```python
from build123d import *

# Parameters (mm, degrees)
SKETCH1_W           = 6
SKETCH1_H           = 6
BOSS_EXTRUDE1_DEPTH = 5
CUT_EXTRUDE5_DEPTH  = 3
CUT_EXTRUDE6_DEPTH  = 3


with BuildPart() as part:
    # Sketch1 → Boss-Extrude1 (new body)
    with BuildSketch(Plane(origin=(0, 0, 0), x_dir=(1, 0, 0), z_dir=(0, 1, 0))):
        Rectangle(SKETCH1_W, SKETCH1_H)
    extrude(amount=BOSS_EXTRUDE1_DEPTH)

    # Sketch8 → Cut-Extrude5 (cut)
    with BuildSketch(Plane.XY.offset(3)):
        Polygon((3, 3), (0, 1.5), (0, 3), (-3, 5), (3, 5), align=None)
    extrude(amount=-CUT_EXTRUDE5_DEPTH, mode=Mode.SUBTRACT)

    # Sketch9 → Cut-Extrude6 (cut)
    with BuildSketch(Plane(origin=(0, 0, -3), x_dir=(-1, 0, 0), z_dir=(0, 0, -1))):
        Polygon((-3, 5), (-3, 3), (0, 1.5), (3, 0), (3, 5), align=None)
    extrude(amount=-CUT_EXTRUDE6_DEPTH, mode=Mode.SUBTRACT)


solid = part.part
```
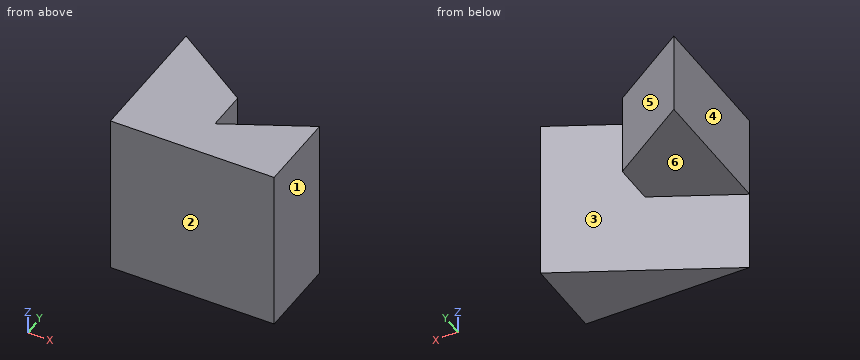
Model file for the job. Use its own axes, mm. Face numbers are marked on the shaded views. A direction names the side the tool comes from. Coordinates: 2 decimals unless noted, no trailing zeros. Order: outer loops, then holes, each group sorted by start corner. A loop starts at its lowest first (then second) coordinate and runs counter-clockwise, first axis right, second up. Notation, with made-up numbers: M 80.5,72 L 101.5,72 A26 cw 101.5,107 Z; hole C 70.25,-7.75 d7. An arc over 180 degrees is marked long. Answer as CSV lines item,"result".
(1) Flat gauge pins, fed straight in: pin 1 (2 mm diameter, centred on x = -0.5, z = 1, fed in from +Y); pin 2 (1.5 mm diameter, centred on y = 4, z = -2.5, fed in from +X). Where does each tip first touch, or does it go through?
Geometry says:
pin 1,"stops at y = 4"
pin 2,"passes through"
(2) Band-saw the part on D-D, the plane y = 3.1. List the corners of the cut face in (x, z).
Geometry says:
outline,"M -3,0 L -0.15,0 L -0.15,3 L -3,3 Z"
(3) Pull direction X, two halves, no side cores. Call the marked faces 1, 2, 3 and 4: +X half, -X half, draft (parallel to the pull), parting line (faces both ways), or undercut.
Geometry says:
face 1,"+X half"
face 2,"draft"
face 3,"undercut"
face 4,"-X half"
(4) Band-saw the part on A-A, the plane y = 2.4. List the corners of the cut face in (x, z).
Geometry says:
outline,"M -3,0 L 0,0 L 0,3 L -3,3 Z; M 1.8,-3 L 3,-3 L 3,3 L 1.8,3 Z"
(5) Band-saw the part on C-C, the plane x = -0.5. List the corners of the cut face in (y, z).
Geometry says:
outline,"M 0,-3 L 1.25,-3 L 1.25,0 L 3.33,0 L 3.33,3 L 0,3 Z"
(6) Band-saw the part on B-B, the plane z = 0.2. List the corners of the cut face in (x, y), then the cut area to 4 significant figures.
Geometry says:
outline,"M -3,0 L 3,0 L 3,3 L 0,1.5 L 0,3 L -3,5 Z"
area,"18.75 mm2"
(7) Wall check: line 1 along Z through (x, y) = (-0.25, 2.05); line 2 along Y through (x, z) = (0, -1); line 3 along Y through (x, z) = (2.5, 2.5). Give the ranges that are in metal, low to high.
Geometry says:
line 1,"z = 0 to 3"
line 2,"y = 0 to 1.5"
line 3,"y = 0 to 2.75"
(8) 3-axis set-ups, long thin cutter, end or side, ignore diameter. For the marked faces 5 and 6: which of +Z, -Z, +X, -X, +Y, -Y reach the whole face in a straight line?
Geometry says:
face 5,"+Z, -Z, +X, +Y"
face 6,"-Z, -X, +Y"
